Part model, mm, in its own coordinate system. A direction names the side the tool comes from. Round coordinates to 2 decimals unless told otherwise and drop trailing zeros. Write each loop counter-clockwise with the first axis right and the second up, starting at its lowest first coordinate (ties: lowest second). Pieces come first, ordered by that corner, then holes. Notation, with made-up numbers: M 21.25,53.5 L 46.25,53.5 A25 cw 46.25,69.5 Z; hole C 81,-7 d8. An arc over 180 degrees is marked long. One line per question, with ' | ' between items. Start each with the question number.
1) Drop flat-ended pins along their axis: pin 1 Ø2 at (x, y) = (15.5, -16.5) entering from -Z; pin 2 Ø3 at (y, z) = (6, 6.5) entering from -X; pin 3 Ø1 at (y, z) = (14.5, 8.5) entering from -X. Give the stop position or say it passes through.
2) Mould opens along X. For faces 1 (the face through (-22, 1, 6)), 2 (the face through (23.846, 7.509, 6.958)), 3 (the face through (-8, 19, 10)) say: pulls with the +X half, pulls with the -X half, needs draft (parallel to the pull), parting line crosses it, or undercut.
3) Saw through at A-A (x = 12.5). List the corners of the cut face in (y, z).
4) Tool access for faces 4 (the face through (-15.726, 15.42, 7.972)), 5 (the face through (-15, -17, 6)): list every direction of +Z, -Z, +X, -X, +Y, -Y with a clear straight run to the whole face (end or side of a thin tool).
5) Wall check: probe 1 along Y at (x, z) = (0, 9.05); probe 2 along X at (y, z) = (-16, 4.3); probe 3 along Y at (x, z) = (-10, 8.4). Give the ranges that are in metal, low to high. Write a range as [from, to].
6) Saw through at B-B (y = -7). List the corners of the cut face in (x, z) (3 decimals).
```python
from build123d import *

# Parameters (mm, degrees)
CYLINDER2777_R               = 1
CYLINDER2777_DEPTH           = 10
CYLINDER2777_PLACEMENT_ANGLE = 45
CYLINDER2779_R               = 1
CYLINDER2779_DEPTH           = 10
CYLINDER2780_R               = 1
CYLINDER2780_DEPTH           = 10
CYLINDER2780_PLACEMENT_ANGLE = 135
CYLINDER2784_R               = 1
CYLINDER2784_DEPTH           = 10
CYLINDER2776_R               = 1
CYLINDER2776_DEPTH           = 10
CYLINDER2776_PLACEMENT_ANGLE = 225
CYLINDER2782_R               = 1
CYLINDER2782_DEPTH           = 10
CYLINDER2775_R               = 1
CYLINDER2775_DEPTH           = 10
CYLINDER2775_PLACEMENT_ANGLE = 45
CYLINDER2774_R               = 1
CYLINDER2774_DEPTH           = 10
CYLINDER2788_R               = 2
CYLINDER2788_DEPTH           = 2
CYLINDER2788_PLACEMENT_ANGLE = 45
CYLINDER2783_R               = 2
CYLINDER2783_DEPTH           = 2
CYLINDER2778_R               = 2
CYLINDER2778_DEPTH           = 2
CYLINDER2778_PLACEMENT_ANGLE = 135
CYLINDER2789_R               = 2
CYLINDER2789_DEPTH           = 2
CYLINDER2785_R               = 2
CYLINDER2785_DEPTH           = 2
CYLINDER2785_PLACEMENT_ANGLE = 225
CYLINDER2786_R               = 2
CYLINDER2786_DEPTH           = 2
CYLINDER2787_R               = 2
CYLINDER2787_DEPTH           = 2
CYLINDER2787_PLACEMENT_ANGLE = 45
CYLINDER2781_R               = 2
CYLINDER2781_DEPTH           = 2
TUBE136_R                    = 25
TUBE136_R_2                  = 20
TUBE136_DEPTH                = 6


with BuildPart() as obj1:
    # Cylinder2777 → Cylinder2777 (new body)
    with BuildSketch(Plane.XY):
        Circle(CYLINDER2777_R)
    extrude(amount=CYLINDER2777_DEPTH)


with BuildPart() as obj1_1:
    # Cylinder2777 placement: moved
    add(obj1.part.moved(Location((-16.263456, 16.263456, 4))).rotate(Axis((-16.263456, 16.263456, 4), (0, 0, 1)), CYLINDER2777_PLACEMENT_ANGLE))


with BuildPart() as obj2:
    # Cylinder2779 → Cylinder2779 (new body)
    with BuildSketch(Plane(origin=(-23, 0, 4), x_dir=(0, 1, 0), z_dir=(0, 0, 1))):
        Circle(CYLINDER2779_R)
    extrude(amount=CYLINDER2779_DEPTH)


with BuildPart() as obj3:
    # Cylinder2780 → Cylinder2780 (new body)
    with BuildSketch(Plane.XY):
        Circle(CYLINDER2780_R)
    extrude(amount=CYLINDER2780_DEPTH)


with BuildPart() as obj3_1:
    # Cylinder2780 placement: moved
    add(obj3.part.moved(Location((-16.263456, -16.263456, 4))).rotate(Axis((-16.263456, -16.263456, 4), (0, 0, 1)), CYLINDER2780_PLACEMENT_ANGLE))


with BuildPart() as obj4:
    # Cylinder2784 → Cylinder2784 (new body)
    with BuildSketch(Plane(origin=(0, -23, 4), x_dir=(-1, 0, 0), z_dir=(0, 0, 1))):
        Circle(CYLINDER2784_R)
    extrude(amount=CYLINDER2784_DEPTH)


with BuildPart() as obj5:
    # Cylinder2776 → Cylinder2776 (new body)
    with BuildSketch(Plane.XY):
        Circle(CYLINDER2776_R)
    extrude(amount=CYLINDER2776_DEPTH)


with BuildPart() as obj5_1:
    # Cylinder2776 placement: moved
    add(obj5.part.moved(Location((16.263456, -16.263456, 4))).rotate(Axis((16.263456, -16.263456, 4), (0, 0, 1)), CYLINDER2776_PLACEMENT_ANGLE))


with BuildPart() as obj6:
    # Cylinder2782 → Cylinder2782 (new body)
    with BuildSketch(Plane(origin=(23, 0, 4), x_dir=(0, -1, 0), z_dir=(0, 0, 1))):
        Circle(CYLINDER2782_R)
    extrude(amount=CYLINDER2782_DEPTH)


with BuildPart() as obj7:
    # Cylinder2775 → Cylinder2775 (new body)
    with BuildSketch(Plane.XY):
        Circle(CYLINDER2775_R)
    extrude(amount=CYLINDER2775_DEPTH)


with BuildPart() as obj7_1:
    # Cylinder2775 placement: moved
    add(obj7.part.moved(Location((16.263456, 16.263456, 4))).rotate(Axis((16.263456, 16.263456, 4), (0, 0, -1)), CYLINDER2775_PLACEMENT_ANGLE))


with BuildPart() as compound1238:
    # Cylinder2774 → Cylinder2774 (new body)
    with BuildSketch(Plane(origin=(0, 23, 4), x_dir=(1, 0, 0), z_dir=(0, 0, 1))):
        Circle(CYLINDER2774_R)
    extrude(amount=CYLINDER2774_DEPTH)

    # Compound1238: union obj1, obj2, obj3, obj4, obj5, obj6, obj7
    add(obj1_1.part)
    add(obj2.part)
    add(obj3_1.part)
    add(obj4.part)
    add(obj5_1.part)
    add(obj6.part)
    add(obj7_1.part)


with BuildPart() as obj8:
    # Cylinder2788 → Cylinder2788 (new body)
    with BuildSketch(Plane.XY):
        Circle(CYLINDER2788_R)
    extrude(amount=CYLINDER2788_DEPTH)


with BuildPart() as obj8_1:
    # Cylinder2788 placement: moved
    add(obj8.part.moved(Location((-16.263456, 16.263456, 4))).rotate(Axis((-16.263456, 16.263456, 4), (0, 0, 1)), CYLINDER2788_PLACEMENT_ANGLE))


with BuildPart() as obj9:
    # Cylinder2783 → Cylinder2783 (new body)
    with BuildSketch(Plane(origin=(-23, 0, 4), x_dir=(0, 1, 0), z_dir=(0, 0, 1))):
        Circle(CYLINDER2783_R)
    extrude(amount=CYLINDER2783_DEPTH)


with BuildPart() as obj10:
    # Cylinder2778 → Cylinder2778 (new body)
    with BuildSketch(Plane.XY):
        Circle(CYLINDER2778_R)
    extrude(amount=CYLINDER2778_DEPTH)


with BuildPart() as obj10_1:
    # Cylinder2778 placement: moved
    add(obj10.part.moved(Location((-16.263456, -16.263456, 4))).rotate(Axis((-16.263456, -16.263456, 4), (0, 0, 1)), CYLINDER2778_PLACEMENT_ANGLE))


with BuildPart() as obj11:
    # Cylinder2789 → Cylinder2789 (new body)
    with BuildSketch(Plane(origin=(0, -23, 4), x_dir=(-1, 0, 0), z_dir=(0, 0, 1))):
        Circle(CYLINDER2789_R)
    extrude(amount=CYLINDER2789_DEPTH)


with BuildPart() as obj12:
    # Cylinder2785 → Cylinder2785 (new body)
    with BuildSketch(Plane.XY):
        Circle(CYLINDER2785_R)
    extrude(amount=CYLINDER2785_DEPTH)


with BuildPart() as obj12_1:
    # Cylinder2785 placement: moved
    add(obj12.part.moved(Location((16.263456, -16.263456, 4))).rotate(Axis((16.263456, -16.263456, 4), (0, 0, 1)), CYLINDER2785_PLACEMENT_ANGLE))


with BuildPart() as obj13:
    # Cylinder2786 → Cylinder2786 (new body)
    with BuildSketch(Plane(origin=(23, 0, 4), x_dir=(0, -1, 0), z_dir=(0, 0, 1))):
        Circle(CYLINDER2786_R)
    extrude(amount=CYLINDER2786_DEPTH)


with BuildPart() as obj14:
    # Cylinder2787 → Cylinder2787 (new body)
    with BuildSketch(Plane.XY):
        Circle(CYLINDER2787_R)
    extrude(amount=CYLINDER2787_DEPTH)


with BuildPart() as obj14_1:
    # Cylinder2787 placement: moved
    add(obj14.part.moved(Location((16.263456, 16.263456, 4))).rotate(Axis((16.263456, 16.263456, 4), (0, 0, -1)), CYLINDER2787_PLACEMENT_ANGLE))


with BuildPart() as compound1239:
    # Cylinder2781 → Cylinder2781 (new body)
    with BuildSketch(Plane(origin=(0, 23, 4), x_dir=(1, 0, 0), z_dir=(0, 0, 1))):
        Circle(CYLINDER2781_R)
    extrude(amount=CYLINDER2781_DEPTH)

    # Compound1239: union obj8, obj9, obj10, obj11, obj12, obj13, obj14
    add(obj8_1.part)
    add(obj9.part)
    add(obj10_1.part)
    add(obj11.part)
    add(obj12_1.part)
    add(obj13.part)
    add(obj14_1.part)


with BuildPart() as cut1046:
    # Tube136 → Tube136 (new body)
    with BuildSketch(Plane.XY.offset(4)):
        Circle(TUBE136_R)
        Circle(TUBE136_R_2, mode=Mode.SUBTRACT)
    extrude(amount=TUBE136_DEPTH)

    # Cut1047: cut Compound1239
    add(compound1239.part, mode=Mode.SUBTRACT)

    # Cut1046: cut Compound1238
    add(compound1238.part, mode=Mode.SUBTRACT)


solid = cut1046.part
```
Answer key:
1) pin 1: stops at z = 6 | pin 2: stops at x = -24.59 | pin 3: stops at x = -20.71
2) face 1: undercut | face 2: parting line crosses it | face 3: needs draft
3) outline: M -21.65,4 L -15.61,4 L -15.61,10 L -21.65,10 Z; M 15.61,4 L 21.65,4 L 21.65,10 L 15.61,10 Z
4) face 4: +Z, -Z | face 5: -Z
5) probe 1: y = [-25, -24], [-22, -20], [20, 22], [24, 25] | probe 2: x = [-19.21, -18.25], [-14.28, -12], [12, 14.28], [18.25, 19.21] | probe 3: y = [-22.91, -17.32], [17.32, 22.91]
6) outline: M -24,4 L -18.735,4 L -18.735,10 L -24,10 Z; M 18.735,4 L 24,4 L 24,10 L 18.735,10 Z
